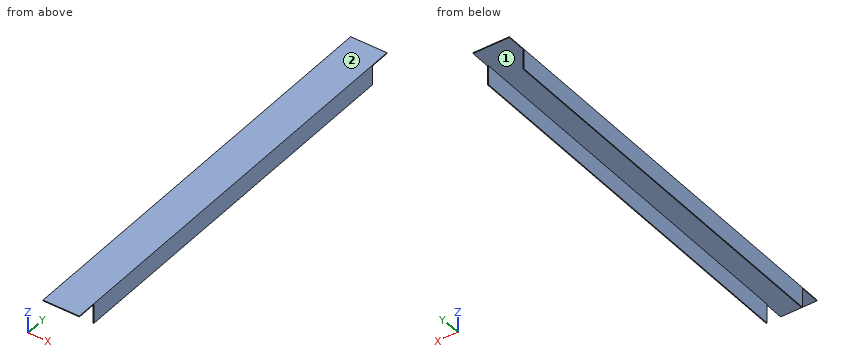
```python
from build123d import *

# Parameters (mm, degrees)
F0_W     = 45
F0_H     = 530
F1_DEPTH = 25
F2_W     = 45
F2_H     = 24
F3_DEPTH = 25
F4_W     = 45
F4_H     = 24
F5_DEPTH = 25
F6_W     = 43
F6_H     = 24
F7_DEPTH = 505.001


with BuildPart() as f1:
    # F0 (on Top) → F1 (new body)
    with BuildSketch(Plane.XY):
        with Locations((22.5, 265)):
            Rectangle(F0_W, F0_H)
    extrude(amount=-F1_DEPTH)

    # F2 (on face) → F3 (cut)
    with BuildSketch(Plane.XZ):
        with Locations((22.5, -13)):
            Rectangle(F2_W, F2_H)
    extrude(amount=-F3_DEPTH, mode=Mode.SUBTRACT)

    # F4 (on face) → F5 (cut)
    with BuildSketch(Plane(origin=(0, 530, 0), x_dir=(-1, 0, 0), z_dir=(0, 1, 0))):
        with Locations((-22.5, -13)):
            Rectangle(F4_W, F4_H)
    extrude(amount=-F5_DEPTH, mode=Mode.SUBTRACT)

    # F6 (on face) → F7 (cut, through all)
    with BuildSketch(Plane(origin=(0, 505, 0), x_dir=(-1, 0, 0), z_dir=(0, 1, 0))):
        with Locations((-22.5, -13)):
            Rectangle(F6_W, F6_H)
    extrude(amount=-F7_DEPTH, mode=Mode.SUBTRACT)


solid = f1.part
```
Here's how the part is built. I have some questions about the finished solid (model axes, mm). Face numbers are marked on the shaded views. Round coordinates to 2 decimals unless told otherwise and drop trailing zeros. Loops run counter-clockwise (first coordinate to the right, second up) from the corner with the lowest first, then second, coordinate; pieces in that order, holes last. Notation, with made-up numbers: (11, 0.25) -> (24, 0.25) arc R23 ccw to (24, 27.25) -> close; hole circle Ø6 at (72.25, 4.5). An arc over 180 degrees is marked (long way). Answer as CSV lines item,"result". Start each with the question number.
1. Imagine slicing it at C-C on x = 33. Write out the boundary of the cut face in (y, z).
2. If we mould it in two halves opening along X, with no side actions, what happens to the marked faces 1 and 2? For each: pulls with the +X half, pulls with the -X half, needs draft (parallel to the pull), parting line crosses it, or undercut.
3. I need wall thicknesses on probe 1 along X at (y, z) = (439.5, -22.25); probe 2 along Z at (x, y) = (38, 35). Which ranges of each line are inside material? Lowest first, please. Write a range as from..to.
4. I'm going to push flat-ended pins straight in: P1, Ø0.5, axis at x = 44.5, z = -17, coming from the +Y side; P2, Ø1.1, axis at x = 44.5, z = -14.5, coming from the -Y side; P3, Ø1, axis at x = 31, y = 109.5, coming from the -Z side. Where does each tip first touch, or does it pass through?
5. Imagine slicing it at A-A on y = 376. Write out the boundary of the cut face in (x, z).
6. Imagine slicing it at B-B on z = -14.75. Write out the boundary of the cut face in (x, y).
Solution:
1,outline,"(0, -1) -> (530, -1) -> (530, 0) -> (0, 0) -> close"
2,face 1,"undercut"
2,face 2,"needs draft"
3,probe 1,"0..1, 44..45"
3,probe 2,"-1..0"
4,P1,"y = 505"
4,P2,"y = 25"
4,P3,"z = -1"
5,outline,"(0, -25) -> (1, -25) -> (1, -1) -> (44, -1) -> (44, -25) -> (45, -25) -> (45, 0) -> (0, 0) -> close"
6,outline,"(0, 25) -> (1, 25) -> (1, 505) -> (0, 505) -> close; (44, 25) -> (45, 25) -> (45, 505) -> (44, 505) -> close"
